Source: CAD feature listing. Evaluate the final solid. Frame: model axes, mm. A direction names the side the tool comes from. Coordinates: 2 decimals unless noted, no trailing zeros. Order: outer loops, then holes, each group sorted by start corner. A loop starts at its lowest first (then second) coordinate and runs counter-clockwise, first axis right, second up.
```python
from build123d import *

# Parameters (mm, degrees)
F1_DEPTH = 16.2179
F2_W     = 11.2395
F2_H     = 2.54
F3_DEPTH = 2.54
F4_DEPTH = 5.2832


with BuildPart() as f1:
    # F0 (on Top) → F1 (new body)
    with BuildSketch(Plane.XY):
        with BuildLine():
            Line((0, 5.0038), (0, 0))
            ThreePointArc((0, 0), (4.0386, -4.0386), (8.0772, 0))
            Line((8.0772, 0), (8.0772, 5.0038))
            ThreePointArc((8.0772, 5.0038), (4.0386, 9.0424), (0, 5.0038))
        make_face()
    extrude(amount=F1_DEPTH)

    # F2 (on face) → F3 (join)
    with BuildSketch(Plane.XY.offset(16.2179)):
        with BuildLine():
            Line((4.0386, -4.0386), (8.0772, -4.0386))
            Line((8.0772, -4.0386), (8.0772, 0))
            ThreePointArc((8.0772, 0), (6.8943214465, -2.8557214465), (4.0386, -4.0386))
        make_face()
        with BuildLine():
            ThreePointArc((4.0386, 9.0424), (6.8943214465, 7.8595214465), (8.0772, 5.0038))
            Line((8.0772, 5.0038), (8.0772, 9.0424))
            Line((8.0772, 9.0424), (4.0386, 9.0424))
        make_face()
        with BuildLine():
            ThreePointArc((0, 0), (1.1828785535, -2.8557214465), (4.0386, -4.0386))
            ThreePointArc((4.0386, -4.0386), (6.8943214465, -2.8557214465), (8.0772, 0))
            Line((8.0772, 0), (8.0772, 5.0038))
            ThreePointArc((8.0772, 5.0038), (6.8943214465, 7.8595214465), (4.0386, 9.0424))
            ThreePointArc((4.0386, 9.0424), (1.1828785535, 7.8595214465), (0, 5.0038))
            Line((0, 5.0038), (0, 0))
        make_face()
        with BuildLine():
            Line((-4.47294, -4.0386), (4.0386, -4.0386))
            ThreePointArc((4.0386, -4.0386), (1.1828785535, -2.8557214465), (0, 0))
            Line((0, 0), (0, 5.0038))
            ThreePointArc((0, 5.0038), (1.1828785535, 7.8595214465), (4.0386, 9.0424))
            Line((4.0386, 9.0424), (-4.47294, 9.0424))
            Line((-4.47294, 9.0424), (-4.47294, 25.80894))
            Line((-4.47294, 25.80894), (-15.71244, 25.80894))
            Line((-15.71244, 25.80894), (-15.71244, -4.0386))
            Line((-15.71244, -4.0386), (-4.47294, -4.0386))
        make_face()
        with Locations((-10.09269, 27.07894)):
            Rectangle(F2_W, F2_H)
    extrude(amount=F3_DEPTH)

    # F2 (on face) → F4 (join)
    with BuildSketch(Plane.XY.offset(16.2179)):
        with Locations((-10.09269, 27.07894)):
            Rectangle(F2_W, F2_H)
    extrude(amount=-F4_DEPTH)


solid = f1.part
```
1. Pin query (flat end, axial travel): P1, Ø1.3, axis at x = 4.5, z = 17, coming from the +Y side; P2, Ø1.5, axis at x = -10.5, y = 8, coming from the -Z side; P3, Ø4, axis at y = 23.5, z = 13.5, coming from the +X side; P4, Ø1.5, axis at x = -4, z = 16.5, coming from the +Y side. Return the tip coordinate at first contact, or that it passes through.
Findings:
P1: stops at y = 9.04
P2: stops at z = 16.22
P3: passes through
P4: stops at y = 28.35
2. Section query A-A on z = 12.5. Return loops of the section in (x, y), plus the area to 3 significant figures.
Findings:
outline: (-15.71, 25.81) - (-4.47, 25.81) - (-4.47, 28.35) - (-15.71, 28.35) - close; (0, 0) arc R4.04 ccw to (8.08, 0) - (8.08, 5) arc R4.04 ccw to (0, 5) - close
area: 120 mm2
3. Section query B-B on y = 1. Return loops of the section in (x, z), plus the area to 3 significant figures.
Findings:
outline: (-15.71, 16.22) - (0, 16.22) - (0, 0) - (8.08, 0) - (8.08, 18.76) - (-15.71, 18.76) - close
area: 191 mm2
4. Ray query, line 1 (Y direction, x = -4.25, z = 17); line 2 (Z direction, x = -6.75, y = 21); line 3 (Y direction, x = -6.5, z = 14.75). Return the intervals inside material, ascending.
Findings:
line 1: y = -4.04 to 9.04
line 2: z = 16.22 to 18.76
line 3: y = 25.81 to 28.35
5. Access query for faces 1 (the face through (-10, 25.809, 14)), 2 (the face through (7, -3, 16.218)), 3 (the face through (0, 3, 8)). Directions: +Z, -Z, +X, -X, +Y, -Y. A direction counts if a zero-diameter tool reaches every point of the face in a straight line with its end or side. Return the directions, or none.
Findings:
face 1: -Z, +X, -X, -Y
face 2: -Z, +X, -Y
face 3: -Z, -X, +Y, -Y
6. Section query C-C on x = 1.5. Return loops of the section in (y, z), plus the area to 3 significant figures.
Findings:
outline: (-4.04, 16.22) - (-3.14, 16.22) - (-3.14, 0) - (8.14, 0) - (8.14, 16.22) - (9.04, 16.22) - (9.04, 18.76) - (-4.04, 18.76) - close
area: 216 mm2
7. Section query D-D on z = 4. Return loops of the section in (x, y).
Findings:
outline: (0, 0) arc R4.04 ccw to (8.08, 0) - (8.08, 5) arc R4.04 ccw to (0, 5) - close
